Source: CAD feature listing. Evaluate the final solid. Frame: model axes, mm. A direction names the side the tool comes from. Give positions to 0.01 mm unless a question says otherwise; leave off trailing zeros. Order: outer loops, then holes, each group sorted by start corner. A loop starts at its lowest first (then second) coordinate and runs counter-clockwise, first axis right, second up. Notation, with made-up numbers: (-36, 3) -> (23, 3) arc R11 cw to (23, 24) -> close; hole circle Ø9 at (-25, -31.75). An arc over 180 degrees is marked (long way). Answer in a Markdown table with one row per item.
```python
from build123d import *

# Parameters (mm, degrees)
SKETCH4_W          = 10
SKETCH4_H          = 24
SKETCH4_W_2        = 5
SKETCH4_H_2        = 12
CUT_EXTRUDE1_DEPTH = 8


with BuildPart() as part:
    # Sketch1 → Revolve1 (revolve)
    with BuildSketch(Plane.XY, mode=Mode.PRIVATE) as revolve1_sk:
        Polygon((0, 0), (0, 2.5), (0.5, 3), (29.5, 3), (30, 2.5), (30, 0), align=None)
    revolve(revolve1_sk.sketch.rotate(Axis((30, 0, 0), (-1, 0, 0)), 270), axis=Axis((30, 0, 0), (-1, 0, 0)))

    # Sketch2 → Cut-Revolve1 (revolve, cut)
    with BuildSketch(Plane.XY, mode=Mode.PRIVATE) as cut_revolve1_sk:
        Polygon((0, 0), (0, 1.5), (0.2705, 1.2295), (6.490147844, 1.2295), (7.2, 0), align=None)
    revolve(cut_revolve1_sk.sketch.rotate(Axis((7.2, 0, 0), (-1, 0, 0)), 270), axis=Axis((7.2, 0, 0), (-1, 0, 0)), mode=Mode.SUBTRACT)

    # Sketch3 → Cut-Revolve2 (revolve, cut)
    with BuildSketch(Plane.XY, mode=Mode.PRIVATE) as cut_revolve2_sk:
        Polygon((22.8, 0), (23.509852156, 1.2295), (29.7295, 1.2295), (30, 1.5), (30, 0), align=None)
    revolve(cut_revolve2_sk.sketch.rotate(Axis((30, 0, 0), (-1, 0, 0)), 270), axis=Axis((30, 0, 0), (-1, 0, 0)), mode=Mode.SUBTRACT)

    # Sketch4 → Cut-Extrude1 (cut)
    with BuildSketch(Plane(origin=(3.5, 0, 0), x_dir=(0, 0, -1), z_dir=(1, 0, 0))):
        Rectangle(SKETCH4_W, SKETCH4_H)
        Rectangle(SKETCH4_W_2, SKETCH4_H_2, mode=Mode.SUBTRACT)
    extrude(amount=CUT_EXTRUDE1_DEPTH, mode=Mode.SUBTRACT)


solid = part.part
```
(1) First-contact query: pin 1 Ø2.5 at (x, y) = (7.5, 0) entering from -Z; pin 2 Ø3 at (x, z) = (12, -2) entering from +Y; pin 3 Ø0.6 at (y, z) = (0, -3) entering from +X. Flat tips, straight axial feed; report the tip coordinate or a pass-through.
A:
| item | result |
|---|---|
| pin 1 | stops at z = -2.5 |
| pin 2 | stops at y = 2.96 |
| pin 3 | stops at x = 29.8 |
(2) Pull-direction query (Z, two-part tool) for faces 4 (the flat face through (7, 0, 2.5)), 5 (the conical face through (7.087, -0.075, 0.181)), 6 (the cylindrical face through (15, 0, -3)); classes: +Z half, -Z half, draft (parallel to the pull), parting line (faces both ways), or undercut.
A:
| item | result |
|---|---|
| face 4 | +Z half |
| face 5 | undercut |
| face 6 | parting line |
(3) Ray query, probe 1 along Y at (x, z) = (1.75, 0); probe 2 along Z at (x, y) = (8.25, 0.55); probe 3 along Z at (x, y) = (27.25, -0.7). Return the intervals inside material, ascending.
A:
| item | result |
|---|---|
| probe 1 | y = -3 to -1.23, 1.23 to 3 |
| probe 2 | z = -2.5 to 2.5 |
| probe 3 | z = -2.92 to -1.01, 1.01 to 2.92 |
(4) Access query for faces 1 (the cylindrical face through (26.66, -1.2, -0.27)), 2 (the flat face through (7, 0, -2.5)), 3 (the cylindrical face through (3.42, -1.2, -0.27)). Directions: +Z, -Z, +X, -X, +Y, -Y. A direction counts if a zero-diameter tool reaches every point of the face in a straight line with its end or side. Return the directions, or none.
A:
| item | result |
|---|---|
| face 1 | +X |
| face 2 | -Z, +Y, -Y |
| face 3 | -X |
(5) Section query A-A (x = 28). Return the cut outline in (y, z), plus the area to 3 significant figures.
A:
| item | result |
|---|---|
| outline | circle Ø6 at (0, 0); hole circle Ø2.46 at (0, 0) |
| area | 23.5 mm^2 |
(6) Section query B-B (x = 20). Return the cut outline in (y, z), plus the area to 3 significant figures.
A:
| item | result |
|---|---|
| outline | circle Ø6 at (0, 0) |
| area | 28.3 mm^2 |
